The listing builds one solid part. Answer for the finished solid, in the listing's coordinates (mm). A direction names the side the tool comes from. Coordinates: 2 decimals unless noted, no trailing zeros. Order: outer loops, then holes, each group sorted by start corner. A loop starts at its lowest first (then second) coordinate and runs counter-clockwise, first axis right, second up. Notation, with made-up numbers: (9.5, -11.5) -> (41.5, -11.5) arc R21 ccw to (41.5, 21.5) -> close; hole circle Ø5 at (81.25, -17). An arc over 180 degrees is marked (long way). Answer in a Markdown table with one row per item.
Autodesk Inventor part; units mm, degrees
ref_plane "Work Plane1" through (-19.25, -0.5, 9.85) normal (0, 0, 1) x (1, 0, 0)
ref_plane "Work Plane2" through (-19.25, -0.5, 12.85) normal (0, 0, 1) x (1, 0, 0)
ref_plane "Work Plane4" through (19.95, -28.3, 9.85) normal (1, 0, 0) x (0, 0, -1)
ref_plane "Work Plane1" through (-19.25, -0.5, 9.85) normal (0, 0, 1) x (1, 0, 0)
sketch "Sketch1" plane through (-19.25, -0.5, 9.85) normal (0, 0, 1) x (1, 0, 0)
  line L0 (-0.695, -27.8) -> (39.2, -27.8)
  line L1 (39.2, -27.8) -> (39.2, 8.9608)
  line L2 (39.2, 8.9608) -> (-0.695, 8.9608)
  line L3 (-0.695, 8.9608) -> (-0.695, -27.8)
  point P0 (19.25, 0.5)
extrude "Extrusion1" add sketch "Sketch1" along normal blind 3
ref_plane "Work Plane2" through (-19.25, -0.5, 12.85) normal (0, 0, 1) x (1, 0, 0)
sketch "Sketch2" plane through (-19.25, -0.5, 12.85) normal (0, 0, 1) x (1, 0, 0)
  line L0 (39.2, -27.8) -> (39.2, 8.9608)
  line L1 (39.2, -27.8) -> (-0.695, -27.8)
  line L2 (-0.695, -27.8) -> (-0.695, 8.9608)
  line L3 (-0.695, 8.9608) -> (39.2, 8.9608)
  line L4 (39.2, 8.9608) -> (39.2, -27.8)
  point P0 (19.25, 0.5)
  point P1 (39.2, 8.9608)
extrude "Extrusion2" add sketch "Sketch2" along normal blind 5
ref_plane "Work Plane4" through (19.95, -28.3, 9.85) normal (1, 0, 0) x (0, 0, -1)
sketch "Sketch3" plane through (19.95, -28.3, 9.85) normal (1, 0, 0) x (0, 0, -1)
  line L0 (0, 0) -> (0, 36.7608)
  line L1 (0, 0) -> (-8, 0)
  line L2 (0, 36.7608) -> (-2, 36.7608)
  line L3 (-2, 36.7608) -> (-2, 0)
  line L4 (-2, 0) -> (0, 0)
  line L5 (0, 0) -> (0, 36.7608)
  point P0 (9.85, 28.3)
  dimension "d4" = 2
extrude "Extrusion3" cut sketch "Sketch3" against normal blind 50
ref_plane "Work Plane3" through (19.95, -28.3, 17.85) normal (1, 0, 0) x (0, 0, -1)
sketch "Sketch4" plane through (19.95, -28.3, 17.85) normal (1, 0, 0) x (0, 0, -1)
  line L0 (6, 0) -> (0, 0)
  line L1 (6, 36.7608) -> (0, 36.7608)
  line L2 (0, 0) -> (1, 0)
  line L3 (1, 0) -> (1, 36.7608)
  line L4 (1, 36.7608) -> (0, 36.7608)
  line L5 (0, 36.7608) -> (0, 0)
  point P0 (17.85, 28.3)
  point P1 (1, 0)
  dimension "d7" = 1
extrude "Extrusion4" cut sketch "Sketch4" against normal blind 50
ref_plane "Work Plane5" through (19.95, -28.3, 11.85) normal (1, 0, 0) x (0, 0, -1)
sketch "Sketch5" plane through (19.95, -28.3, 11.85) normal (1, 0, 0) x (0, 0, -1)
  line L0 (-5, 36.7608) -> (-5, 0)
  line L1 (0, 0) -> (0, 36.7608)
  line L2 (-5, 36.7608) -> (0, 36.7608)
  line L3 (0, 36.7608) -> (0, 0)
  line L4 (0, 0) -> (-5, 0)
  line L5 (-5, 0) -> (-5, 36.7608)
  point P0 (11.85, 28.3)
extrude "Extrusion5" add sketch "Sketch5" along normal blind 7
ref_plane "Work Plane6" through (-19.945, -28.3, 11.85) normal (0, 0, -1) x (-1, 0, 0)
sketch "Sketch6" plane through (-19.945, -28.3, 11.85) normal (0, 0, -1) x (-1, 0, 0)
  line L0 (-46.895, 0) -> (-46.895, 36.7608)
  line L1 (-46.895, 27.8459) -> (-40.895, 27.8459)
  line L2 (-40.895, 27.8459) -> (-40.895, 11.8459)
  line L3 (-40.895, 11.8459) -> (-46.895, 11.8459)
  line L4 (-46.895, 11.8459) -> (-46.895, 27.8459)
  point P0 (-19.945, 28.3)
  dimension "d12" = 6
  dimension "d13" = 16
extrude "Extrusion6" add sketch "Sketch6" along normal blind 22.875
sketch "Sketch7" plane through (20.95, -0.4541, 11.85) normal (0, 1, 0) x (1, 0, 0)
  arc A0 (5.4164, 8.2173) -> (5.4164, 5.6327) centre (3.7611, 6.925) ccw
  circle A1 centre (3.7611, 6.925) radius 2.5
  arc A2 (5.4164, 18.0673) -> (5.4164, 15.4827) centre (3.7611, 16.775) ccw
  circle A3 centre (3.7611, 16.775) radius 2.5
  point P0 (-20.95, 11.85)
  dimension "d16" = 5
  dimension "d17" = 5
extrude "Extrusion7" cut sketch "Sketch7" against normal blind 22.875
ref_plane "Work Plane7" through (26.95, -28.3, 11.85) normal (1, 0, 0) x (0, 0, -1)
sketch "Sketch8" plane through (26.95, -28.3, 11.85) normal (1, 0, 0) x (0, 0, -1)
  line L0 (0, 11.8459) -> (22.875, 11.8459)
  line L1 (22.875, 27.8459) -> (22.875, 11.8459)
  line L2 (0, 11.8459) -> (22.875, 11.8459)
  line L3 (22.875, 11.8459) -> (22.875, 16.8459)
  line L4 (22.875, 16.8459) -> (0, 16.8459)
  line L5 (0, 16.8459) -> (0, 11.8459)
  point P0 (11.85, 28.3)
  dimension "d20" = 5
extrude "Extrusion8" cut sketch "Sketch8" against normal blind 6.7
ref_plane "Work Plane8" through (-19.945, -28.3, 11.85) normal (-1, 0, 0) x (0, 0, 1)
sketch "Sketch9" plane through (-19.945, -28.3, 11.85) normal (-1, 0, 0) x (0, 0, 1)
  line L0 (0, 36.7608) -> (0, 0)
  line L1 (5, 0) -> (0, 0)
  line L2 (0, 36.7608) -> (5, 36.7608)
  line L3 (5, 36.7608) -> (5, 0)
  line L4 (5, 0) -> (0, 0)
  line L5 (0, 0) -> (0, 36.7608)
  point P0 (-11.85, 28.3)
extrude "Extrusion9" add sketch "Sketch9" along normal blind 7
ref_plane "Work Plane10" through (26.95, -0.4541, 11.85) normal (0, 0, -1) x (-1, 0, 0)
sketch "Sketch11" plane through (26.95, -0.4541, 11.85) normal (0, 0, -1) x (-1, 0, 0)
  line L0 (53.895, -27.8459) -> (53.895, 8.9148)
  line L1 (53.895, 0) -> (47.895, 0)
  line L2 (47.895, 0) -> (47.895, -11)
  line L3 (47.895, -11) -> (53.895, -11)
  line L4 (53.895, -11) -> (53.895, 0)
  point P0 (26.95, 0.4541)
  dimension "d25" = 6
extrude "Extrusion10" add sketch "Sketch11" along normal blind 22.875
sketch "Sketch12" plane through (-26.945, -0.4541, 11.85) normal (0, 1, 0) x (1, 0, 0)
  arc A0 (0.5786, 15.4827) -> (0.5786, 18.0673) centre (2.2339, 16.775) ccw
  circle A1 centre (2.2339, 16.775) radius 2.5
  arc A2 (0.5786, 5.6327) -> (0.5786, 8.2173) centre (2.2339, 6.925) ccw
  circle A3 centre (2.2339, 6.925) radius 2.5
  point P0 (26.945, 11.85)
  dimension "d28" = 5
  dimension "d29" = 5
extrude "Extrusion11" cut sketch "Sketch12" against normal blind 22.875
ref_plane "Work Plane11" through (-26.945, -28.3, 11.85) normal (-1, 0, 0) x (0, 0, 1)
sketch "Sketch13" plane through (-26.945, -28.3, 11.85) normal (-1, 0, 0) x (0, 0, 1)
  line L0 (0, 16.8459) -> (0, 27.8459)
  line L1 (5, 36.7608) -> (0, 36.7608)
  line L2 (0, 27.8459) -> (5, 27.8459)
  line L3 (5, 27.8459) -> (5, 36.7608)
  line L4 (5, 36.7608) -> (0, 36.7608)
  line L5 (0, 36.7608) -> (0, 27.8459)
  point P0 (-11.85, 28.3)
extrude "Extrusion12" cut sketch "Sketch13" against normal blind 67.325
ref_plane "Work Plane9" through (26.95, -28.3, 11.85) normal (0, -1, 0) x (1, 0, 0)
sketch "Sketch14" plane through (26.95, -28.3, 11.85) normal (0, -1, 0) x (1, 0, 0)
  line L0 (0, 5) -> (0, 0)
  line L1 (0, 5) -> (-53.895, 5)
  line L2 (0, 0) -> (-53.895, 0)
  line L3 (-53.895, 0) -> (-53.895, 5)
  line L4 (-53.895, 5) -> (0, 5)
  line L5 (0, 5) -> (0, 0)
  point P0 (-26.95, -11.85)
extrude "Extrusion13" add sketch "Sketch14" along normal blind 5
ref_plane "Work Plane12" through (26.95, -11.4541, 11.85) normal (0, 0, -1) x (-1, 0, 0)
sketch "Sketch15" plane through (26.95, -11.4541, 11.85) normal (0, 0, -1) x (-1, 0, 0)
  line L0 (53.895, -21.8459) -> (0, -21.8459)
  line L1 (53.895, 11) -> (53.895, -21.8459)
  line L2 (0, -21.8459) -> (53.895, -21.8459)
  line L3 (53.895, -21.8459) -> (53.895, -17.8459)
  line L4 (53.895, -17.8459) -> (0, -17.8459)
  line L5 (0, -17.8459) -> (0, -21.8459)
  point P0 (26.95, 11.4541)
  dimension "d36" = 4
extrude "Extrusion14" add sketch "Sketch15" along normal blind 22.4625
ref_plane "Work Plane13" through (-26.945, -29.3, 11.85) normal (0, 1, 0) x (1, 0, 0)
sketch "Sketch16" plane through (-26.945, -29.3, 11.85) normal (0, 1, 0) x (1, 0, 0)
  line L0 (53.895, 0) -> (53.895, 22.4625)
  line L1 (0, 0) -> (0, 22.4625)
  line L2 (53.895, 0) -> (0, 0)
  line L3 (0, 0) -> (0, 1)
  line L4 (0, 1) -> (53.895, 1)
  line L5 (53.895, 1) -> (53.895, 0)
  point P0 (26.945, 11.85)
  point P1 (53.895, 1)
  dimension "d39" = 1
extrude "Extrusion15" add sketch "Sketch16" along normal blind 30
ref_plane "Work Plane14" through (26.95, -28.3, 11.85) normal (1, 0, 0) x (0, 0, -1)
sketch "Sketch17" plane through (26.95, -28.3, 11.85) normal (1, 0, 0) x (0, 0, -1)
  line L0 (0, 29) -> (1, 29)
  line L1 (5.8126, 27.8459) -> (1, 27.8459)
  line L2 (0, 29) -> (1, 29)
  line L3 (1, 29) -> (1, 27.8459)
  line L4 (1, 27.8459) -> (0, 27.8459)
  line L5 (0, 27.8459) -> (0, 29)
  point P0 (11.85, 28.3)
extrude "Extrusion16" cut sketch "Sketch17" against normal blind 100
sketch "Sketch19" plane through (26.95, -33.3, 11.85) normal (0, -1, 0) x (1, 0, 0)
  circle A0 centre (-16.85, -11.85) radius 5
  circle A1 centre (-16.85, -11.85) radius 1.5
  point P0 (-26.95, -11.85)
  dimension "d47" = 10
  dimension "d50" = 3
extrude "Extrusion20" cut sketch "Sketch19" against normal blind 10 contours A1
sketch "Sketch20" plane through (26.95, -33.3, 11.85) normal (0, -1, 0) x (1, 0, 0)
  line L0 (-53.895, -22.4625) -> (0, -22.4625)
  line L1 (-53.895, 5) -> (-53.895, -22.4625)
  line L2 (0, -22.4625) -> (-53.895, -22.4625)
  line L3 (-53.895, -22.4625) -> (-53.895, 5)
  line L4 (-53.895, 5) -> (0, 5)
  line L5 (0, 5) -> (0, -22.4625)
  point P0 (-26.95, -11.85)
extrude "Extrusion21" add sketch "Sketch20" along normal blind 2
sketch "Sketch21" plane through (-26.945, -29.3, -10.6125) normal (0, 1, 0) x (1, 0, 0)
  circle A0 centre (37.045, -10.6125) radius 1.5
  circle A1 centre (37.045, -10.6125) radius 1.5
  point P0 (26.945, -10.6125)
extrude "Extrusion22" cut sketch "Sketch21" against normal blind 10
sketch "Sketch22" plane through (-26.945, -29.3, -10.6125) normal (0, 1, 0) x (1, 0, 0)
  circle A0 centre (37.045, -10.6125) radius 1.5
  circle A1 centre (37.045, -10.6125) radius 2.5
  point P0 (26.945, -10.6125)
  dimension "d59" = 5
extrude "Extrusion23" cut sketch "Sketch22" against normal blind 2
sketch "Sketch23" plane through (-19.945, -28.3, -11.025) normal (0, 0, -1) x (-1, 0, 0)
  line L0 (-46.895, 27.8459) -> (-46.895, 16.8459)
  line L1 (-46.895, 27.8459) -> (-48.895, 27.8459)
  line L2 (-48.895, 27.8459) -> (-48.895, 16.8459)
  line L3 (-48.895, 16.8459) -> (-46.895, 16.8459)
  line L4 (-46.895, 16.8459) -> (-46.895, 27.8459)
  line L5 (7, 16.8459) -> (7, 27.8459)
  line L6 (7, 27.8459) -> (9, 27.8459)
  line L7 (9, 27.8459) -> (9, 16.8459)
  line L8 (9, 16.8459) -> (7, 16.8459)
  line L9 (7, 16.8459) -> (7, 27.8459)
  point P0 (-19.945, 28.3)
  dimension "d62" = 2
  dimension "d63" = 2
extrude "Extrusion24" add sketch "Sketch23" against normal up to surface (27.875 mm away)
sketch "Sketch24" plane through (-20.945, -0.4541, 10.85) normal (0, 1, 0) x (1, 0, 0)
  arc A0 (47.895, 7.0374) -> (47.895, 4.8126) centre (45.6561, 5.925) ccw
  circle A1 centre (45.6561, 5.925) radius 1.6
  arc A2 (47.895, 16.8874) -> (47.895, 14.6626) centre (45.6561, 15.775) ccw
  circle A3 centre (45.6561, 15.775) radius 1.6
  circle A4 centre (45.6561, 5.925) radius 2.5
  circle A5 centre (45.6561, 15.775) radius 2.5
  point P0 (20.945, 10.85)
  point P1 (47.895, 4.8126)
  dimension "d66" = 3.2
  dimension "d67" = 3.2
extrude "Extrusion25" add sketch "Sketch24" against normal up to surface (11 mm away)
sketch "Sketch25" plane through (-20.945, -0.4541, 10.85) normal (0, 1, 0) x (1, 0, 0)
  arc A0 (-6, 4.8025) -> (-6, 7.0475) centre (-3.7661, 5.925) ccw
  circle A1 centre (-3.7661, 5.925) radius 1.6
  arc A2 (-6, 14.6525) -> (-6, 16.8975) centre (-3.7661, 15.775) ccw
  circle A3 centre (-3.7661, 15.775) radius 1.6
  circle A4 centre (-3.7661, 15.775) radius 2.5
  circle A5 centre (-3.7661, 5.925) radius 2.5
  point P0 (20.945, 10.85)
  point P1 (-6, 7.0475)
  dimension "d70" = 3.2
  dimension "d71" = 3.2
  dimension "d72" = 5
  dimension "d73" = 5
extrude "Extrusion26" add sketch "Sketch25" against normal up to surface (11 mm away)
properties part number "MG996RServoHolder" material "钢"
(1) Find the intervals of material crossed by line 1 along X through (y, z) = (-9, -1.75) (3 decimals); line 2 along Y through (x, z) = (23, -5); line 3 along Z through (x, y) = (-20, -17.5), in increasing order. Write a range as from..to.
Check values:
| item | result |
|---|---|
| line 1 | -28.945..-20.945, 20.95..28.95 |
| line 2 | -35.3..-29.3, -11.45..-0.45 |
| line 3 | 10.85..16.85 |
(2) For a pull along X with two mould halves and no side action, classify faces 6 (the flat face through (-20.945, -6, 0)), 7 (the flat face through (0, -35.3, 3)), 8 (the flat face through (-28.945, -6, 3)), 9 (the flat face through (20.95, -6, 0)) as released by +X, released by -X, zero draft, split by the parting line, or undercut.
Check values:
| item | result |
|---|---|
| face 6 | undercut |
| face 7 | zero draft |
| face 8 | released by -X |
| face 9 | undercut |
(3) A cutting plane is placed at B-B, the plane x = 10.1. Determine the outline of the cut face in (y, z), then the cut area to 3 significant figures.
Check values:
| item | result |
|---|---|
| outline | (-35.3, -10.61) -> (-29.3, -10.61) -> (-29.3, -2.5) -> (-31.3, -2.5) -> (-31.3, -1.5) -> (-35.3, -1.5) -> close; (-35.3, 1.5) -> (-31.3, 1.5) -> (-31.3, 2.5) -> (-29.3, 2.5) -> (-29.3, 10.85) -> (-0.45, 10.85) -> (-0.45, 16.85) -> (-35.3, 16.85) -> close |
| area | 316 mm² |
(4) Which of the six approach directions +Z, -Z, +X, -X, +Y, -Y give full straight-line access (tool end or side, diameter ignored) to faces 1 (the flat face through (-25, -6, -11.025)), 2 (the cylindrical face through (7.6, -30.3, -0.1)), 3 (the flat face through (0, -15, 10.85)), 4 (the flat face through (0, -29.3, 0)), 5 (the flat face through (26.95, -31, 9))?
Check values:
| item | result |
|---|---|
| face 1 | -Z, +X, -X, +Y, -Y |
| face 2 | +Y |
| face 3 | -Z |
| face 4 | -Z, +X, -X |
| face 5 | +Z, -Z, +X, -Y |
(5) A cutting plane is placed at D-D, the plane x = -24.5. Count the separate pieces of the cut face and the enclosed holes in it, then the cut area to 3 significant figures.
Check values:
| item | result |
|---|---|
| separate pieces | 3 |
| enclosed holes | 0 |
| area | 509 mm² |
(6) A cutting plane is placed at A-A, the plane z = 0. Determine the outline of the cut face in (x, y) (3 decimals).
Check values:
| item | result |
|---|---|
| outline | (-28.945, -11.454) -> (-20.945, -11.454) -> (-20.945, -0.454) -> (-28.945, -0.454) -> close; (-26.945, -35.3) -> (8.6, -35.3) -> (8.6, -31.3) -> (7.6, -31.3) -> (7.6, -29.3) -> (-26.945, -29.3) -> close; (11.6, -35.3) -> (26.95, -35.3) -> (26.95, -29.3) -> (12.6, -29.3) -> (12.6, -31.3) -> (11.6, -31.3) -> close; (20.95, -11.454) -> (28.95, -11.454) -> (28.95, -0.454) -> (20.95, -0.454) -> close |
(7) Flat-ended cylindrical pins translate along their axes: pin 1 (1.8 mm diameter, centred on x = 7, y = -33.5, fed in from -Z); pin 2 (2 mm diameter, centred on x = 10, z = 10.5, fed in from +Y); pin 3 (14.5 mm diameter, centred on x = 5.5, y = -10.5, fed in from -Z); pin 4 (5 mm diameter, centred on x = -14, z = 4, fed in from +Y). Find the tip coordinate at first contact, or state that the pin passes through.
Check values:
| item | result |
|---|---|
| pin 1 | z = -10.61 |
| pin 2 | y = -0.45 |
| pin 3 | z = 10.85 |
| pin 4 | y = -29.3 |
(8) A cutting plane is placed at C-C, the plane z = 4.25. Determine the outline of the cut face in (x, y) (3 decimals), then the cut area to 3 significant figures.
Check values:
| item | result |
|---|---|
| outline | (-28.945, -11.454) -> (-26.162, -11.454) -> (-26.162, -0.454) -> (-28.945, -0.454) -> close; (-26.945, -35.3) -> (26.95, -35.3) -> (26.95, -29.3) -> (-26.945, -29.3) -> close; (-23.26, -11.454) -> (-20.945, -11.454) -> (-20.945, -0.454) -> (-23.26, -0.454) -> close; (20.95, -11.454) -> (23.26, -11.454) -> (23.26, -0.454) -> (20.95, -0.454) -> close; (26.162, -11.454) -> (28.95, -11.454) -> (28.95, -0.454) -> (26.162, -0.454) -> close |
| area | 436 mm² |
